Study the drawing (mm; zero at the part's minimum x, y, z) and answer. A direction names the side the tool comes from. Give positions to 0.01 mm unless a question says otherwise; leave off trailing zeros. Loops run counter-clockwise (first coordinate to the right, second up) from the corner with the lowest first, then second, coordinate; pieces in that order, holes last. Notation, with made-up numbers: (48, 56.25) - (87, 56.25) arc R26 cw to (87, 93.25) - close; hole circle Ø10 at (41.5, -39.75). An arc over 180 degrees is marked (long way). Write item = value, one per line. Start each with the question number.
1) Which of the six approach directions +Z, -Z, +X, -X, +Y, -Y give full straight-line access (tool end or side, diameter ignored) to the marked faces 1 and 2?
2) The part is cut by section C-C on z = 15. Write down the section's boundary in (x, y).
3) The part is cut by section A-A on x = 2.5. Write down the section's boundary in (y, z) (1 decimal).
4) The part is cut by section D-D on z = 10.5. Write down the section's boundary in (x, y), plus the area to 3 significant figures.
5) Consider probe 1 along Y at (x, z) = (17.25, 15); probe 2 along Z at (x, y) = (10.75, 11.5) (1 decimal); probe 3 along X at (y, z) = (10.5, 18.25). Determine where each line is inside the solid, lowest interval first.
6) The part is cut by section B-B on y = 12.25. Write down the section's boundary in (x, z) (1 decimal).
7) The mould has two halves that part along Y. Classify the marked faces 3, 4 and 5: +Y half, -Y half, draft (parallel to the pull), parting line (faces both ways), or undercut.
8) Flat-ended cylindrical pins translate along their axes: P1, Ø6, axis at x = 6, z = 4.5, coming from the -Y side; P2, Ø3, axis at x = 9, y = 23.5, coming from the -Z side; P3, Ø2, axis at x = 11.5, z = 25, coming from the +Y side. Find the tip coordinate at first contact, or state that the pin passes through.
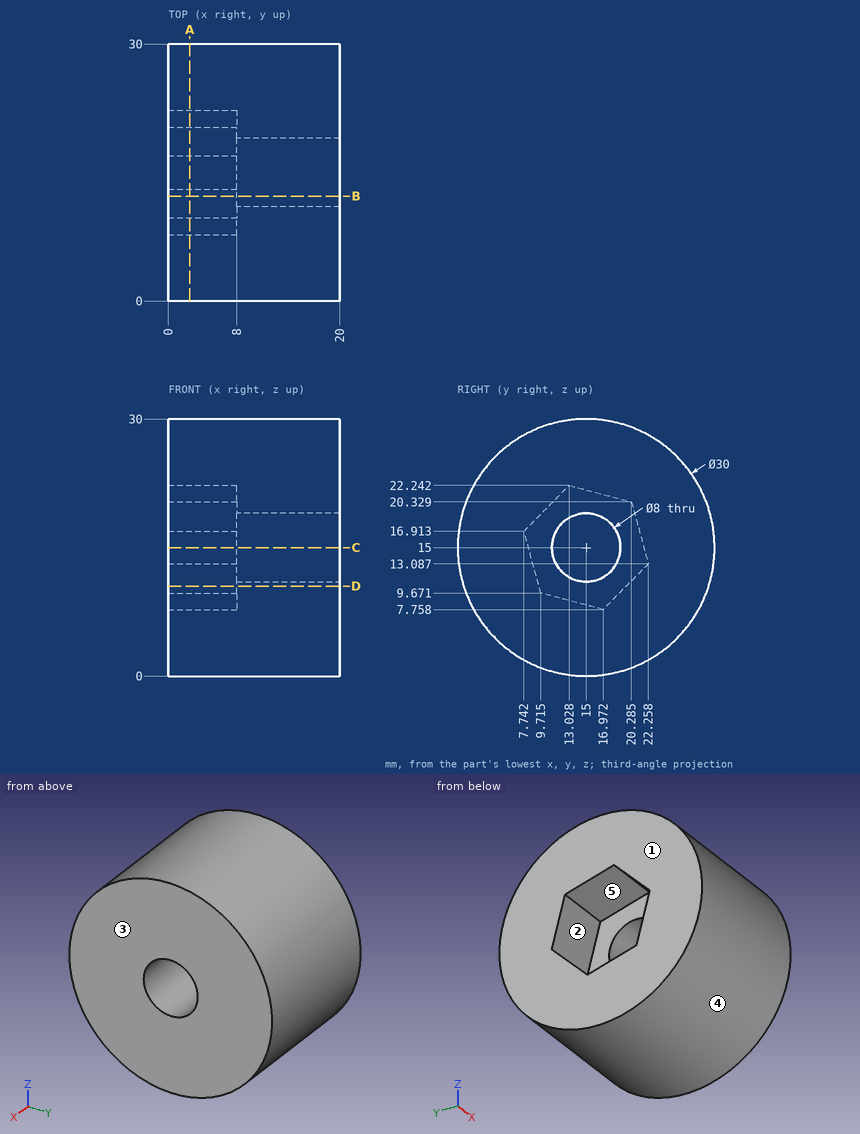
Answer below:
q1.face_1 = +Z, -Z, -X, +Y, -Y
q1.face_2 = -X
q2.outline = (0, 0) - (20, 0) - (20, 11) - (8, 11) - (8, 8.26) - (0, 8.26) - close; (0, 21.74) - (8, 21.74) - (8, 19) - (20, 19) - (20, 30) - (0, 30) - close
q3.outline = circle Ø30 at (15, 15); hole (7.7, 16.9) - (9.7, 9.7) - (17, 7.8) - (22.3, 13.1) - (20.3, 20.3) - (13, 22.2) - close
q4.outline = (0, 0.69) - (20, 0.69) - (20, 29.31) - (0, 29.31) - (0, 19.69) - (8, 19.69) - (8, 9.49) - (0, 9.49) - close
q4.area = 491 mm2
q5.probe_1 = 0 to 11, 19 to 30
q5.probe_2 = 0.4 to 13.1, 16.9 to 29.6
q5.probe_3 = 8 to 20
q6.outline = (0, 0.3) - (20, 0.3) - (20, 12.1) - (8, 12.1) - (8, 9) - (0, 9) - close; (0, 21.5) - (8, 21.5) - (8, 17.9) - (20, 17.9) - (20, 29.7) - (0, 29.7) - close
q7.face_3 = draft
q7.face_4 = parting line
q7.face_5 = undercut
q8.P1 = 2.01
q8.P2 = 1.73
q8.P3 = 27
